For this review, take the finished solid that the model builds, in its own axes (mm). Face numbers are marked on the shaded views. A direction names the side the tool comes from. Give positions to 0.01 mm unless a question says otherwise; leave off trailing zeros. Loops run counter-clockwise (first coordinate to the right, second up) from the corner with the lowest first, then second, coordinate; pieces in that order, holes last. Notation, with made-up numbers: (7.25, 7.25) -> (16.25, 7.25) arc R29 cw to (16.25, 30.25) -> close; hole circle Ø3 at (86, -16). An arc over 180 degrees is marked (long way). One line per question, with ' | ' between items. Start each with the question number.
(1) Consider section D-D (y = -18.5). Write out the cut boundary in (x, z).
(2) Wall thickness on probe 1 along Z at (x, y) = (29.5, -24.5); probe 2 along X at (y, z) = (-26, 30.5); probe 3 along Z at (x, y) = (0, -1.2): over which ranges is each line inside the solid? List them lowest first.
(3) Consider section B-B (x = 0). Write out the cut boundary in (y, z) (3 decimals), and give its area (3 significant figures).
(4) Draft analysis for pull direction Z (two halves, no side actions). For the marked faces 3, 4 and 5, state which applies: +Z half, -Z half, draft (parallel to the pull), parting line (faces both ways), or undercut.
(5) Consider section A-A (z = 24.5). Write out the cut boundary in (x, y) (3 decimals), and give its area (3 significant figures).
(6) Insertion check: P1, Ø1, axis at x = 4.5, y = -2, coming from the -Z side; P2, Ø0.8, axis at x = 39, z = 19.5, coming from the +Y side. Each pin has a flat end and moves straight along its axis. Give the tip position at first contact, or say it passes through.
(7) Consider section C-C (x = 13). Write out the cut boundary in (y, z) (3 decimals).
(8) Tool access review of the marked faces 1 and 2: name each direction out of +Z, -Z, +X, -X, +Y, -Y from which nothing blocks a thin tool from reaching the whole face with its end or side.
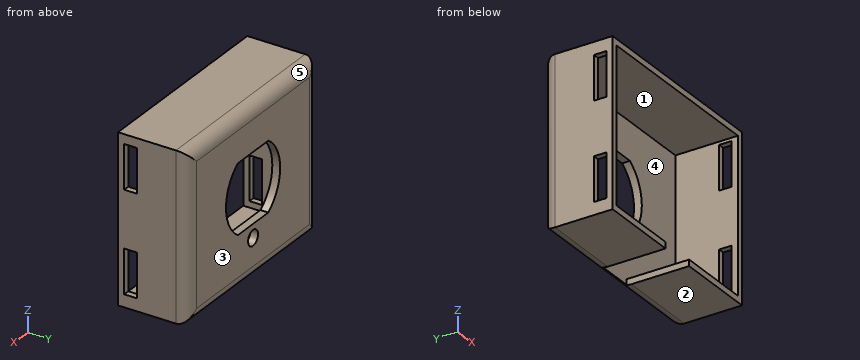
from build123d import *

# Parameters (mm, degrees)
F0_W         = 80.772
F0_H         = 67.3239192
F0_R         = 3.0975808
F1_DEPTH     = 3.175
F2_W         = 80.772
F2_H         = 67.3239192
F2_W_2       = 75.692
F2_H_2       = 62.2439192
F3_DEPTH     = 25.4
F4_W         = 14.732
F4_H         = 25.4
F5_DEPTH     = 25.4
F6_W         = 5.08
F6_H         = 17.78
F7_DEPTH     = 25.4
F8_W         = 5.08
F8_H         = 17.78
F9_DEPTH     = 25.4
F10_T1_DEPTH = 106.172
F10_T3_DEPTH = 92.7239192


# Not quite as in the source:
# - a fillet or chamfer that OpenCascade refuses, or shapes differently, is made with other operations: its cross-section is extruded or revolved along the edge and cut away or added


with BuildPart() as f1:
    # F0 (on Front) → F1 (new body)
    with BuildSketch(Plane.XZ):
        Rectangle(F0_W, F0_H)
        with Locations((0, -17.5051212)):
            Circle(F0_R, mode=Mode.SUBTRACT)
        with BuildLine():
            Line((9.4944692, -12.0580404), (-9.4944692, -12.0580404))
            ThreePointArc((-9.4944692, -12.0580404), (-16.8909981247, 1.9119596), (-9.4944692, 15.8819596))
            Line((-9.4944692, 15.8819596), (9.4944692, 15.8819596))
            ThreePointArc((9.4944692, 15.8819596), (16.8909981247, 1.9119596), (9.4944692, -12.0580404))
        make_face(mode=Mode.SUBTRACT)
    extrude(amount=F1_DEPTH)

    # F2 (on face) → F3 (join)
    with BuildSketch(Plane.XZ.offset(3.175)):
        Rectangle(F2_W, F2_H)
        Rectangle(F2_W_2, F2_H_2, mode=Mode.SUBTRACT)
    extrude(amount=F3_DEPTH)

    # F4 (on face) → F5 (cut)
    with BuildSketch(Plane.XY.offset(-31.1219596)):
        with Locations((0, -15.875)):
            Rectangle(F4_W, F4_H)
    extrude(amount=-F5_DEPTH, mode=Mode.SUBTRACT)

    # F6 (on face) → F7 (cut)
    with BuildSketch(Plane.YZ.offset(40.386)):
        with Locations((-23.495, 20.9619596)):
            Rectangle(F6_W, F6_H)
        with Locations((-23.495, -19.6919596)):
            Rectangle(F6_W, F6_H)
    extrude(amount=-F7_DEPTH, mode=Mode.SUBTRACT)

    # F8 (on face) → F9 (cut)
    with BuildSketch(Plane(origin=(-40.386, 0, 0), x_dir=(0, -1, 0), z_dir=(-1, 0, 0))):
        with Locations((23.495, 19.6919596)):
            Rectangle(F8_W, F8_H)
        with Locations((23.495, -19.6919596)):
            Rectangle(F8_W, F8_H)
    extrude(amount=-F9_DEPTH, mode=Mode.SUBTRACT)

    # F10: fillet of radius 5.08 on 4 edges, made by hand

    # F10_s2 → F10_t1 (cut)
    with BuildSketch(Plane.YZ.offset(-53.086)):
        with BuildLine():
            ThreePointArc((0, 28.5819596), (-1.4878975516, 32.1740620484), (-5.08, 33.6619596))
            Line((-5.08, 33.6619596), (0, 33.6619596))
            Line((0, 33.6619596), (0, 28.5819596))
        make_face()
        with BuildLine():
            ThreePointArc((-5.08, -33.6619596), (-1.4878975516, -32.1740620484), (0, -28.5819596))
            Line((0, -28.5819596), (0, -33.6619596))
            Line((0, -33.6619596), (-5.08, -33.6619596))
        make_face()
    extrude(amount=F10_T1_DEPTH, mode=Mode.SUBTRACT)

    # F10_s4 → F10_t3 (cut)
    with BuildSketch(Plane.XY.offset(-46.3619596)):
        with BuildLine():
            ThreePointArc((-35.306, 0), (-38.8981024484, -1.4878975516), (-40.386, -5.08))
            Line((-40.386, -5.08), (-40.386, 0))
            Line((-40.386, 0), (-35.306, 0))
        make_face()
        with BuildLine():
            ThreePointArc((40.386, -5.08), (38.8981024484, -1.4878975516), (35.306, 0))
            Line((35.306, 0), (40.386, 0))
            Line((40.386, 0), (40.386, -5.08))
        make_face()
    extrude(amount=F10_T3_DEPTH, mode=Mode.SUBTRACT)


solid = f1.part
A:
1) outline: (-40.39, -33.66) -> (-7.37, -33.66) -> (-7.37, -31.12) -> (-37.85, -31.12) -> (-37.85, 31.12) -> (37.85, 31.12) -> (37.85, -31.12) -> (7.37, -31.12) -> (7.37, -33.66) -> (40.39, -33.66) -> (40.39, 33.66) -> (-40.39, 33.66) -> close
2) probe 1: z = -33.66 to -31.12, 31.12 to 33.66 | probe 2: x = -40.39 to -37.85, 37.85 to 40.39 | probe 3: z = -31.86 to -20.6, -14.41 to -12.06, 15.88 to 31.86
3) outline: (-28.575, 31.122) -> (-3.175, 31.122) -> (-3.175, 15.882) -> (0, 15.882) -> (0, 28.582) arc R5.08 ccw to (-5.08, 33.662) -> (-28.575, 33.662) -> close; (-3.175, -33.291) arc R5.08 ccw to (0, -28.582) -> (0, -20.603) -> (-3.175, -20.603) -> close; (-3.175, -14.408) -> (0, -14.408) -> (0, -12.058) -> (-3.175, -12.058) -> close | area: 159 mm^2
4) face 3: draft | face 4: undercut | face 5: +Z half
5) outline: (-40.386, -28.575) -> (-37.846, -28.575) -> (-37.846, -26.035) -> (-40.386, -26.035) -> close; (-40.386, -20.955) -> (-37.846, -20.955) -> (-37.846, -3.175) -> (37.846, -3.175) -> (37.846, -20.955) -> (40.386, -20.955) -> (40.386, -5.08) arc R5.08 ccw to (35.306, 0) -> (-35.306, 0) arc R5.08 ccw to (-40.386, -5.08) -> close; (37.846, -28.575) -> (40.386, -28.575) -> (40.386, -26.035) -> (37.846, -26.035) -> close | area: 349 mm^2
6) P1: stops at z = -32.96 | P2: stops at y = -1.21
7) outline: (-28.575, -33.662) -> (-5.08, -33.662) arc R5.08 ccw to (0, -28.582) -> (0, -8.873) -> (-3.175, -8.873) -> (-3.175, -31.122) -> (-28.575, -31.122) -> close; (-28.575, 31.122) -> (-3.175, 31.122) -> (-3.175, 12.696) -> (0, 12.696) -> (0, 28.582) arc R5.08 ccw to (-5.08, 33.662) -> (-28.575, 33.662) -> close
8) face 1: -Y | face 2: -Z, +X, -X, +Y, -Y
